Model file for the job. Use its own axes, mm. A direction names the side the tool comes from. Give positions to 0.01 mm unless a question says otherwise; leave off trailing zeros. Write each loop counter-clockwise with the first axis right and the second up, starting at its lowest first coordinate (ties: lowest second). Pieces come first, ordered by that corner, then holes. Notation, with made-up numbers: (50, 5) - (92, 5) arc R33 cw to (92, 34) - close; hole circle Ø1 at (30.5, 48.5). An arc over 180 degrees is marked (long way). Use CSV: the item, a comma, the result in double quotes.
from build123d import *

# Parameters (mm, degrees)
BOSS_EXTRUDE1_DEPTH             = 1.5
BOSS_EXTRUDE1_DEPTH_BACK        = 1.5
SKETCH3_R                       = 2
SKETCH4_R                       = 3
CUT_EXTRUDE1_DEPTH              = 3.5
TAP_DRILL_FOR_M4X0_7_TAP1_D     = 3.3
TAP_DRILL_FOR_M4X0_7_TAP1_DEPTH = 10
TAP_DRILL_FOR_M4X0_7_TAP1_TIP   = 0.991420021
TAP_DRILL_FOR_M5X0_8_TAP1_D     = 4.2
TAP_DRILL_FOR_M5X0_8_TAP1_DEPTH = 10
TAP_DRILL_FOR_M5X0_8_TAP1_TIP   = 1.2618073
CUT_EXTRUDE2_DEPTH              = 3
FILLET1_R                       = 2.5
SKETCH12_R                      = 2.75
CUT_EXTRUDE3_DEPTH              = 3
TAP_DRILL_FOR_M3X0_5_TAP2_D     = 2.5
TAP_DRILL_FOR_M3X0_5_TAP2_DEPTH = 10
TAP_DRILL_FOR_M3X0_5_TAP2_TIP   = 0.751075774


with BuildPart() as part:
    # Sketch2 → Revolve1 (revolve)
    with BuildSketch(Plane(origin=(0, 0, 0), x_dir=(1, 0, 0), z_dir=(0, 1, 0)), mode=Mode.PRIVATE) as revolve1_sk:
        Polygon((-77.5, 0), (-77.5, 6), (-51.5, 6), (-51.5, 16), (-48, 16), (-48, 26), (-35, 26), (-35, 25.9), (-3.25, 25.9), (-3.25, 26), (0, 26), (0, 25), (104, 25), (104, 24), (108, 24), (108, 8), (109, 8), (109, 4), (124, 4), (124, 0), align=None)
    revolve(revolve1_sk.sketch.rotate(Axis((-131.1939937, 0, 0), (1, 0, 0)), 180), axis=Axis((-131.1939937, 0, 0), (1, 0, 0)))

    # Sketch3 → Boss-Extrude1 (add, two sides: drawn at the far end of the back side and taken through both)
    with BuildSketch(Plane(origin=(0, 6, 0), x_dir=(1, 0, 0), z_dir=(0, 1, 0)).offset(-BOSS_EXTRUDE1_DEPTH_BACK)):
        with BuildLine():
            Line((-56.5, 2), (-72.5, 2))
            ThreePointArc((-72.5, 2), (-71.085786438, 1.414213562), (-70.5, 0))
            ThreePointArc((-70.5, 0), (-71.085786438, -1.414213562), (-72.5, -2))
            Line((-72.5, -2), (-56.5, -2))
            ThreePointArc((-56.5, -2), (-58.5, 0), (-56.5, 2))
        make_face()
        with Locations((-72.5, 0)):
            Circle(SKETCH3_R)
        with Locations((-56.5, 0)):
            Circle(SKETCH3_R)
    extrude(amount=BOSS_EXTRUDE1_DEPTH + BOSS_EXTRUDE1_DEPTH_BACK)

    # Sketch4 → Cut-Extrude1 (cut)
    with BuildSketch(Plane.ZY.offset(77.5)):
        Circle(SKETCH4_R)
    extrude(amount=-CUT_EXTRUDE1_DEPTH, mode=Mode.SUBTRACT)

    # Tap Drill for M4x0.7 Tap1
    with Locations(Plane.ZY.offset(74)):
        with Locations((0, 0)):
            Hole(TAP_DRILL_FOR_M4X0_7_TAP1_D / 2, depth=TAP_DRILL_FOR_M4X0_7_TAP1_DEPTH)
            with Locations((0, 0, -(TAP_DRILL_FOR_M4X0_7_TAP1_DEPTH + TAP_DRILL_FOR_M4X0_7_TAP1_TIP / 2))):  # 118° drill point
                Cone(0, TAP_DRILL_FOR_M4X0_7_TAP1_D / 2, TAP_DRILL_FOR_M4X0_7_TAP1_TIP, mode=Mode.SUBTRACT)

    # Tap Drill for M5x0.8 Tap1
    with Locations(Plane.ZY.offset(48)):
        with Locations((0, 22.5), (14.142135624, 14.142135624), (22.5, 0), (14.142135624, -14.142135624), (0, -22.5), (-14.142135624, -14.142135624), (-22.5, 0), (-14.142135624, 14.142135624)):
            Hole(TAP_DRILL_FOR_M5X0_8_TAP1_D / 2, depth=TAP_DRILL_FOR_M5X0_8_TAP1_DEPTH)
            with Locations((0, 0, -(TAP_DRILL_FOR_M5X0_8_TAP1_DEPTH + TAP_DRILL_FOR_M5X0_8_TAP1_TIP / 2))):  # 118° drill point
                Cone(0, TAP_DRILL_FOR_M5X0_8_TAP1_D / 2, TAP_DRILL_FOR_M5X0_8_TAP1_TIP, mode=Mode.SUBTRACT)

    # Sketch13 → Cut-Extrude2 (cut)
    with BuildSketch(Plane(origin=(108, 0, 0), x_dir=(0, 0, -1), z_dir=(1, 0, 0))):
        Polygon((-16.970562748, -2.828427125), (-25.455844123, -11.313708499), (-11.313708499, -25.455844123), (-2.828427125, -16.970562748), align=None)
    extrude(amount=-CUT_EXTRUDE2_DEPTH, mode=Mode.SUBTRACT)

    # Fillet1
    fillet1_edges = [part.edges().sort_by_distance(p)[0] for p in [
        (106.5, -16.970562748, 2.828427125),
        (106.5, -2.828427125, 16.970562748),
    ]]
    fillet(fillet1_edges, radius=FILLET1_R)

    # Sketch12 → Cut-Extrude3 (cut)
    with BuildSketch(Plane(origin=(108, 0, 0), x_dir=(0, 0, -1), z_dir=(1, 0, 0))):
        with Locations((-6.759588899, 19.088490195)):
            Circle(SKETCH12_R)
        with Locations((19.957510196, 3.429327453)):
            Circle(SKETCH12_R)
        with Locations((0, -20.25)):
            Circle(SKETCH12_R)
    extrude(amount=-CUT_EXTRUDE3_DEPTH, mode=Mode.SUBTRACT)

    # Tap Drill for M3x0.5 Tap2
    with Locations(Plane(origin=(105, 0, 0), x_dir=(0, 0, -1), z_dir=(1, 0, 0))):
        with Locations((-6.759588899, 19.088490195), (19.957510196, 3.429327453), (0, -20.25)):
            Hole(TAP_DRILL_FOR_M3X0_5_TAP2_D / 2, depth=TAP_DRILL_FOR_M3X0_5_TAP2_DEPTH)
            with Locations((0, 0, -(TAP_DRILL_FOR_M3X0_5_TAP2_DEPTH + TAP_DRILL_FOR_M3X0_5_TAP2_TIP / 2))):  # 118° drill point
                Cone(0, TAP_DRILL_FOR_M3X0_5_TAP2_D / 2, TAP_DRILL_FOR_M3X0_5_TAP2_TIP, mode=Mode.SUBTRACT)


solid = part.part
(1) Flat gauge pins, fed straight in: P1, Ø10, axis at y = -15.5, z = -5, coming from the +X side; P2, Ø4.5, axis at x = -60.5, z = -0.5, coming from the +Y side; P3, Ø6, axis at x = 20, y = 6.5, coming from the +Z side. Where does each tip first touch, or does it go through?
Checked values:
P1,"stops at x = 108"
P2,"stops at y = 7.5"
P3,"stops at z = 24.75"
(2) Saw through at A-A, the plane x = 7. List the corners of the cut face in (y, z), then the cut area to 3 significant figures.
Checked values:
outline,"circle Ø50 at (0, 0)"
area,"1,960 mm^2"
(3) Pull direction Z, two halves, no side cores. Call faces 6 (the face through (105, 2, -21)), 7 (the face through (108.51, 7.81, -1.73)), 8 (the face through (-51.5, 0, -7)): released by +Z, released by -Z, zero draft, split by the parting line, or undercut.
Checked values:
face 6,"undercut"
face 7,"split by the parting line"
face 8,"zero draft"
(4) 3-axis set-ups, long thin cutter, end or side, ignore diameter. For faces 1 (the face through (106.52, 4.26, -22.58)), 2 (the face through (106.52, -20.64, 6.5)), 3 (the face through (-65, 7.5, 0)), 4 (the face through (-42.93, 24.27, -1.13)), 5 (the face through (-77.5, -3, -1)): which of +Z, -Z, +X, -X, +Y, -Y reach the whole face in a straight line?
Checked values:
face 1,"+X"
face 2,"+Z, +X"
face 3,"+Z, -Z, -X, +Y"
face 4,"-X"
face 5,"+Z, -Z, -X, +Y, -Y"
(5) Wall check: probe 1 along Y at (x, z) = (-40.75, 0); probe 2 along Y at (x, z) = (-67, 0); probe 3 along X at (y, z) = (17.5, -12). Give the ranges that are in metal, low to high. Write a range as [from, to].
Checked values:
probe 1,"y = [-26, -24.6], [-20.4, 20.4], [24.6, 26]"
probe 2,"y = [-6, -1.65], [1.65, 7.5]"
probe 3,"x = [-48, 108]"
